Geometry: final body of the model. Coordinates: model frame, mm. A direction names the side the tool comes from. Give positions to 0.01 mm unless a question says otherwise; leave off trailing zeros. Write each loop counter-clockwise with the first axis right and the second up, starting at its lowest first coordinate (ties: lowest second). Pieces come first, ordered by that corner, then holes. Notation, with made-up numbers: M 11,49 L 47,49 A25 ccw 47,65 Z; hole C 82,-23.75 d2. An arc over 180 degrees is marked long. Use a Markdown table: item, result. Add a question column.
1) Line query: line 1 (Z direction, x = -7, y = 14.5); line 2 (Y direction, x = 0, z = 154); line 3 (Z direction, x = -5, y = -3.5). Output: solid intervals per line, ascending.
2) Section A-A on z = 219.71. Return the cut outline in (x, y).
3) Pin query (flat end, axial travel): pin 1 (1.7 mm diameter, centred on y = -7, z = 16, fed in from +X); pin 2 (5 mm diameter, centred on y = 4, z = 48.5, fed in from -X); pin 3 (1 mm diameter, centred on x = -0.5, z = 181.5, fed in from -Y). Return the tip coordinate at first contact, or that it passes through.
4) Section B-B on x = 0. Return the cut outline in (y, z).
5) Set-up query: faces 1 (the cylindrical face through (7.504, -18.768, 220.04)), 2 (the cylindrical face through (1.08, -4.88, 102.51)), 3 (the flat face through (0, -8, 9)). Return all of +Z, -Z, +X, -X, +Y, -Y with unobstructed straight access to the full face (end or side cutting, diameter ignored); none if empty.
6) Draft query along Z for faces 4 (the flat face through (8, 0, 202.21)), 5 (the flat face through (6, 20, 220)), 6 (the cylindrical face through (6.48, -18.57, 201.21)). Return one class per face: +Z half, -Z half, draft (parallel to the pull), parting line (faces both ways), or undercut.
7) Section C-C on y = 2. Return the cut outline in (x, z).
8) Section D-D on z = 145.5. Return the cut outline in (x, y).
```python
from build123d import *

# Parameters (mm, degrees)
SKETCH2_R           = 10
BOSS_EXTRUDE1_DEPTH = 199.71
CUT_EXTRUDE2_DEPTH  = 4.55
SKETCH5_W           = 32.5
SKETCH5_H           = 40
BOSS_EXTRUDE2_DEPTH = 40
SKETCH10_W          = 35
SKETCH10_H          = 35
CUT_EXTRUDE3_DEPTH  = 30
SKETCH11_W          = 20
SKETCH11_H          = 15
CUT_EXTRUDE4_DEPTH  = 2.5
FILLET1_R           = 5
SKETCH12_R          = 5
CUT_EXTRUDE5_DEPTH  = 199.71
SKETCH2_2_R         = 10
CUT_EXTRUDE6_DEPTH  = 8
BOSS_EXTRUDE3_DEPTH = 1
SKETCH16_R          = 15
CUT_EXTRUDE7_DEPTH  = 10


with BuildPart() as part:
    # Sketch2 → Boss-Extrude1 (new body)
    with BuildSketch(Plane.XY):
        Circle(SKETCH2_R)
    extrude(amount=BOSS_EXTRUDE1_DEPTH)

    # Sketch4 → Cut-Extrude2 (cut)
    with BuildSketch(Plane(origin=(0, -10, 0), x_dir=(-1, 0, 0), z_dir=(0, -1, 0))):
        with BuildLine():
            Line((-4.55, -23.788408852), (-4.55, -4.788408852))
            Line((-4.55, -4.788408852), (4.55, -4.788408852))
            Line((4.55, -4.788408852), (4.55, -23.788408852))
            ThreePointArc((4.55, -23.788408852), (6.2, -28), (4.55, -32.211591148))
            Line((4.55, -32.211591148), (4.55, -51.211591148))
            Line((4.55, -51.211591148), (-4.55, -51.211591148))
            Line((-4.55, -51.211591148), (-4.55, -32.211591148))
            ThreePointArc((-4.55, -32.211591148), (-6.2, -28), (-4.55, -23.788408852))
        make_face()
    extrude(amount=-CUT_EXTRUDE2_DEPTH, mode=Mode.SUBTRACT)

    # Sketch5 → Boss-Extrude2 (add)
    with BuildSketch(Plane.XY.offset(199.71)):
        with Locations((6.25, 0)):
            Rectangle(SKETCH5_W, SKETCH5_H)
    extrude(amount=BOSS_EXTRUDE2_DEPTH)

    # Sketch10 → Cut-Extrude3 (cut)
    with BuildSketch(Plane(origin=(22.5, 0, 0), x_dir=(0, 0, -1), z_dir=(1, 0, 0))):
        with Locations((-219.71, 0)):
            Rectangle(SKETCH10_W, SKETCH10_H)
    extrude(amount=-CUT_EXTRUDE3_DEPTH, mode=Mode.SUBTRACT)

    # Sketch11 → Cut-Extrude4 (cut)
    with BuildSketch(Plane(origin=(-7.5, 0, 0), x_dir=(0, 0, -1), z_dir=(1, 0, 0))):
        with Locations((-219.71, 0)):
            Rectangle(SKETCH11_W, SKETCH11_H)
    extrude(amount=-CUT_EXTRUDE4_DEPTH, mode=Mode.SUBTRACT)

    # Fillet1
    fillet1_edges = [part.edges().sort_by_distance(p)[0] for p in [
        (6.25, 20, 199.71),
        (6.25, -20, 199.71),
        (6.25, 20, 239.71),
        (6.25, -20, 239.71),
    ]]
    fillet(fillet1_edges, radius=FILLET1_R)

    # Sketch12 → Cut-Extrude5 (cut)
    with BuildSketch(Plane(origin=(0, 0, 0), x_dir=(-1, 0, 0), z_dir=(0, 0, -1))):
        Circle(SKETCH12_R)
    extrude(amount=-CUT_EXTRUDE5_DEPTH, mode=Mode.SUBTRACT)

    # Sketch2<2> → Cut-Extrude6 (cut)
    with BuildSketch(Plane.XY):
        with Locations(Location((0, 0, 0), (0, 0, 180))):
            Circle(SKETCH2_2_R)
    extrude(amount=CUT_EXTRUDE6_DEPTH, mode=Mode.SUBTRACT)

    # Sketch15 → Boss-Extrude3 (add)
    with BuildSketch(Plane(origin=(0, 0, 8), x_dir=(-1, 0, 0), z_dir=(0, 0, -1))):
        with BuildLine():
            Line((4.55, -8.904914374), (4.55, -5.45))
            Line((4.55, -5.45), (-4.55, -5.45))
            Line((-4.55, -5.45), (-4.55, -8.904914374))
            ThreePointArc((-4.55, -8.904914374), (0, -10), (4.55, -8.904914374))
        make_face()
    extrude(amount=-BOSS_EXTRUDE3_DEPTH)

    # Sketch16 → Cut-Extrude7 (cut)
    with BuildSketch(Plane.XZ.offset(20)):
        with Locations((22.5, 219.71)):
            Circle(SKETCH16_R)
    extrude(amount=-CUT_EXTRUDE7_DEPTH, mode=Mode.SUBTRACT)


solid = part.part
```
Found:
| question | item | result |
|---|---|---|
| 1 | line 1 | 199.71 to 202.21, 237.21 to 239.71 |
| 1 | line 2 | -10 to -5, 5 to 10 |
| 1 | line 3 | 8 to 202.21, 237.21 to 239.71 |
| 2 | outline | M -10,-20 L 7.5,-20 L 7.5,-17.5 L -7.5,-17.5 L -7.5,-7.5 L -10,-7.5 Z; M -10,7.5 L -7.5,7.5 L -7.5,17.5 L 22.5,17.5 L 22.5,20 L -10,20 Z |
| 3 | pin 1 | x = 7.89 |
| 3 | pin 2 | x = -9.89 |
| 3 | pin 3 | y = -10 |
| 4 | outline | M -20,204.71 A5 ccw -15,199.71 L -10,199.71 L -10,51.21 L -5.45,51.21 L -5.45,9 L -10,9 L -10,8 L -5,8 L -5,199.71 L 5,199.71 L 5,8 L 10,8 L 10,199.71 L 15,199.71 A5 ccw 20,204.71 L 20,234.71 A5 ccw 15,239.71 L -15,239.71 A5 ccw -20,234.71 Z; hole M -17.5,202.21 L 17.5,202.21 L 17.5,237.21 L -17.5,237.21 Z |
| 5 | face 1 | +X, -Y |
| 5 | face 2 | -Z |
| 5 | face 3 | -Y |
| 6 | face 4 | undercut |
| 6 | face 5 | draft |
| 6 | face 6 | -Z half |
| 7 | outline | M -10,199.71 L -9.8,199.71 L -9.8,8 L -4.58,8 L -4.58,199.71 L 4.58,199.71 L 4.58,8 L 9.8,8 L 9.8,199.71 L 22.5,199.71 L 22.5,202.21 L -7.5,202.21 L -7.5,209.71 L -10,209.71 Z; M -10,229.71 L -7.5,229.71 L -7.5,237.21 L 22.5,237.21 L 22.5,239.71 L -10,239.71 Z |
| 8 | outline | C 0,0 d20; hole C 0,0 d10 |
